Geometry check sheet. Reference: the model listing, model coordinates, mm. A direction names the side the tool comes from. Coordinates: 2 decimals unless noted, no trailing zeros. Loops run counter-clockwise (first coordinate to the right, second up) from the corner with the lowest first, then second, coordinate; pieces in that order, holes last. Notation, with made-up numbers: M -22.75,31 L 28.25,31 A33 cw 28.25,66 Z; hole C -9,20 d6. An arc over 180 degrees is marked long. Use CSV: the item, a comma, the result in double quotes.
Autodesk Inventor part; units mm, degrees
ref_plane "Start Plane" through (0, 0, 0) normal (0, 0, 1) x (1, 0, 0)
ref_plane "End Plane" through (0, 0, 50.8) normal (0, 0, 1) x (1, 0, 0)
ref_plane "YZ Plane" through (0, 0, 0) normal (1, 0, 0) x (0, 1, 0)
ref_plane "Start Plane" through (0, 0, 0) normal (0, 0, 1) x (1, 0, 0)
ref_plane "End Plane" through (0, 0, 50.8) normal (0, 0, 1) x (1, 0, 0)
sketch "Sketch1" plane through (0, 0, 0) normal (0, 0, 1) x (1, 0, 0)
  line L0 (-19.05, 19.05) -> (19.05, 19.05)
  line L1 (19.05, 19.05) -> (19.05, -19.05)
  line L2 (19.05, -19.05) -> (-19.05, -19.05)
  line L3 (-19.05, -19.05) -> (-19.05, 19.05)
  line L4 (15.875, 15.875) -> (-15.875, 15.875)
  line L5 (-15.875, 15.875) -> (-15.875, -15.875)
  line L6 (-15.875, -15.875) -> (15.875, -15.875)
  line L7 (15.875, -15.875) -> (15.875, 15.875)
  point P0 (0, 0)
  point P1 (0, 19.05)
  point P2 (-19.05, 0)
  dimension "width" = 38.1
  dimension "d1" = 3.175
extrude "Body" add sketch "Sketch1" along normal up to surface (50.8 mm away) from surface at 0
sketch "Sketch4" plane through (0, 0, 0) normal (0, 0, 1) x (1, 0, 0)
  line L0 (0, 0) -> (10, 0)
ref_plane "Work Plane4" through (0, 0, 0) normal (0, -1, 0) x (1, 0, 0)
sketch "Sketch5" plane through (0, 0, 0) normal (0, -1, 0) x (1, 0, 0)
  line L0 (-26.67, 0) -> (26.67, 0)
  line L1 (-26.67, 50.8) -> (26.67, 50.8)
  dimension "d9" = 50.8
equation "\"G_OFFSET_START\" = 0"
equation "\"G_OFFSET_END\" = 0"
equation "\"d5\" = length + G_OFFSET_END"
equation "\"G_L\" = d9"
properties part number "1.5x1.5x.125 Tube"
1. Release check for a two-part mould opening along X. For faces 1 (the flat face through (19.05, 0, 25)), 2 (the flat face through (0, 15.875, 25)), 3 (the flat face through (0, 19.05, 25)), 4 (the flat face through (-19.05, 0, 25)) record: +X half, -X half, draft (parallel to the pull), parting line (faces both ways), or undercut.
The answers:
face 1,"+X half"
face 2,"undercut"
face 3,"draft"
face 4,"-X half"
2. Section check A-A, the plane z = 21. Record the cut outline in (x, y) (3 decimals).
The answers:
outline,"M -19.05,-19.05 L 19.05,-19.05 L 19.05,19.05 L -19.05,19.05 Z; hole M -15.875,-15.875 L 15.875,-15.875 L 15.875,15.875 L -15.875,15.875 Z"
3. Section check B-B, the plane x = -12. Record the cut outline in (y, z) (3 decimals), plus the area to 3 significant figures.
The answers:
outline,"M -19.05,0 L -15.875,0 L -15.875,50.8 L -19.05,50.8 Z; M 15.875,0 L 19.05,0 L 19.05,50.8 L 15.875,50.8 Z"
area,"323 mm^2"
4. Thickness scan on line 1 (X direction, y = -10, z = 13) (3 decimals). Record the ranges inside material, lowest first. Write a range as [from, to].
The answers:
line 1,"[-19.05, -15.875], [15.875, 19.05]"
5. Set-up check for faces 5 (the flat face through (-15.875, 0, 25)), 6 (the flat face through (-17, 0, 0)): record each of +Z, -Z, +X, -X, +Y, -Y from which the full face is reachable in a straight line by a thin tool's end or side.
The answers:
face 5,"+Z, -Z"
face 6,"-Z, +X, -X, +Y, -Y"
